The listing builds one solid part. Answer for the finished solid, in the listing's coordinates (mm). A direction names the side the tool comes from. Give positions to 0.01 mm unless a question says otherwise; leave off trailing zeros. Write each loop counter-clockwise with the first axis right and the second up, starting at its lowest first coordinate (ties: lowest second). Pieces come first, ordered by that corner, then holes. Notation, with made-up numbers: (80, 15) -> (113, 15) arc R20 ccw to (113, 37) -> close; hole circle Ø9 at (25.5, -20.5). An arc over 180 degrees is marked (long way). Put each result on its own line as item: value. Start each with the question number.
1) Flat-ended cylindrical pins translate along their axes: pin 1 Ø0.9 at (y, z) = (58227.5, 5.5) entering from -X; pin 2 Ø0.9 at (x, y) = (41556, 58228.5) entering from +Z; pin 3 Ø0.6 at (x, y) = (41573, 58227) entering from +Z; pin 4 Ø1.8 at (x, z) = (41574.36, 9.5) entering from +Y. Find the tip coordinate at first contact, or state that the pin passes through.
2) Find the intervals of material crossed by line 1 along Z through (x, y) = (41560, 58227.6); line 2 along X through (y, z) = (58226.9, 3.5); line 3 along Z through (x, y) = (41569, 58228.6), in increasing order. Write a range as from..to.
3) A cutting plane is placed at B-B (y = 58229.05). Give the number of separate pieces and of enclosed holes in the cut face, then the cut area to 3 significant figures.
4) For faces 5 (the flat face through (41550, 58228, 7.5)), 6 (the flat face through (41566, 58228, 13.5)), 7 (the cylindrical face through (41544.114, 58227.979, -2.502)), 8 (the flat face through (41560, 58226.458, -7)), determine the directions among +Z, -Z, +X, -X, +Y, -Y from which every point of the face is accessible in a straight line to the end or side of a thin tool.
5) A cutting plane is placed at C-C (z = 1). Write down the section's boundary in (x, y).
6) A cutting plane is placed at A-A (x = 41571). Write down the section's boundary in (y, z), then the cut area to 3 significant figures.
7) A cutting plane is placed at D-D (z = 10). Write down the section's boundary in (x, y).
8) For a pull along X with two mould halves and no side action, classify faces 1 (the cylindrical face through (41547.25, 58227.98, 8.43)), 2 (the flat face through (41544.361, 58228, 1)), 3 (the cylindrical face through (41556.8, 58228, 14)), 4 (the flat face through (41569, 58228, 7.5)) as released by +X, released by -X, zero draft, split by the parting line, or undercut.
from build123d import *

# Parameters (mm, degrees)
CROQUIS1_R                 = 1.5
SALIENTE_EXTRUIR1_DEPTH    = 3
S_LIDO_MOVER_COPIAR1_ANGLE = 90


with BuildPart() as part:
    # Croquis1 → Saliente-Extruir1 (new body)
    with BuildSketch(Plane.XY):
        with BuildLine():
            Line((41558.361281649, 58239.957618209), (41574.361281649, 58239.957618209))
            ThreePointArc((41574.361281649, 58239.957618209), (41576.482601992, 58239.078938552), (41577.361281649, 58236.957618209))
            Line((41577.361281649, 58236.957618209), (41577.361281649, 58218.957618209))
            ThreePointArc((41577.361281649, 58218.957618209), (41576.482601992, 58216.836297865), (41574.361281649, 58215.957618209))
            Line((41574.361281649, 58215.957618209), (41558.361281649, 58215.957618209))
            ThreePointArc((41558.361281649, 58215.957618209), (41556.861281649, 58215.457618209), (41555.361281649, 58215.957618209))
            Line((41555.361281649, 58215.957618209), (41545.861281649, 58216.957618209))
            ThreePointArc((41545.861281649, 58216.957618209), (41542.614003581, 58219.151790828), (41543.438204726, 58222.983226695))
            ThreePointArc((41543.438204726, 58222.983226695), (41544.120880282, 58223.971337158), (41544.361281649, 58225.148033968))
            Line((41544.361281649, 58225.148033968), (41544.361281649, 58230.767202449))
            ThreePointArc((41544.361281649, 58230.767202449), (41544.120880282, 58231.94389926), (41543.438204726, 58232.932009723))
            ThreePointArc((41543.438204726, 58232.932009723), (41542.614003581, 58236.76344559), (41545.86128165, 58238.957618209))
            Line((41545.86128165, 58238.957618209), (41555.361281649, 58239.957618209))
            ThreePointArc((41555.361281649, 58239.957618209), (41556.861281649, 58240.457618209), (41558.361281649, 58239.957618209))
        make_face()
        with Locations((41545.861281649, 58235.457618209)):
            Circle(CROQUIS1_R, mode=Mode.SUBTRACT)
        with Locations((41545.861281649, 58219.857618209)):
            Circle(CROQUIS1_R, mode=Mode.SUBTRACT)
        with Locations((41574.361281649, 58219.957618209)):
            Circle(CROQUIS1_R, mode=Mode.SUBTRACT)
        with Locations((41574.361281649, 58235.957618209)):
            Circle(CROQUIS1_R, mode=Mode.SUBTRACT)
        Polygon((41551.361281649, 58236.957618209), (41566.361281649, 58236.957618209), (41566.361281649, 58233.957618209), (41572.361281649, 58233.957618209), (41572.361281649, 58230.957618209), (41574.361281649, 58230.957618209), (41574.361281649, 58225.957618209), (41572.361281649, 58225.957618209), (41572.361281649, 58221.457618208), (41549.261281649, 58221.457618208), (41549.261281649, 58233.957618209), (41551.361281649, 58233.957618209), align=None, mode=Mode.SUBTRACT)
    extrude(amount=SALIENTE_EXTRUIR1_DEPTH)


with BuildPart() as part_1:
    # Sólido-Mover/Copiar1: moved
    add(part.part.rotate(Axis((0, 58227.957618209, 1.5), (1, 0, 0)), S_LIDO_MOVER_COPIAR1_ANGLE))


solid = part_1.part
Reply:
1. pin 1: stops at x = 41543.87
1. pin 2: stops at z = 13.97
1. pin 3: stops at z = 13.5
1. pin 4: passes through
2. line 1: z = -10.5..-5, 10.5..13.5
2. line 2: x = 41544.36..41549.26, 41574.36..41577.36
2. line 3: z = -10.5..-5, 7.5..13.5
3. separate pieces: 1
3. enclosed holes: 5
3. area: 424 mm2
4. face 5: +Y, -Y
4. face 6: +Z, +X, +Y, -Y
4. face 7: -X, +Y, -Y
4. face 8: +Z, -Z, +X, -X, -Y
5. outline: (41544.36, 58226.46) -> (41549.26, 58226.46) -> (41549.26, 58229.46) -> (41544.36, 58229.46) -> close; (41574.36, 58226.46) -> (41577.36, 58226.46) -> (41577.36, 58229.46) -> (41574.36, 58229.46) -> close
6. outline: (58226.46, -10.5) -> (58229.46, -10.5) -> (58229.46, -5) -> (58226.46, -5) -> close; (58226.46, 7.5) -> (58229.46, 7.5) -> (58229.46, 13.5) -> (58226.46, 13.5) -> close
6. area: 34.5 mm2
7. outline: (41542.51, 58226.46) -> (41544.74, 58226.46) -> (41544.74, 58229.46) -> (41542.51, 58229.46) -> close; (41546.98, 58226.46) -> (41551.36, 58226.46) -> (41551.36, 58229.46) -> (41546.98, 58229.46) -> close; (41566.36, 58226.46) -> (41572.95, 58226.46) -> (41572.95, 58229.46) -> (41566.36, 58229.46) -> close; (41575.78, 58226.46) -> (41577.36, 58226.46) -> (41577.36, 58229.46) -> (41575.78, 58229.46) -> close
8. face 1: undercut
8. face 2: released by -X
8. face 3: split by the parting line
8. face 4: undercut
